```python
from build123d import *

# Parameters (mm, degrees)
SKETCH1_R           = 80
SKETCH1_R_2         = 1.1
SKETCH1_R_3         = 3.7
BOSS_EXTRUDE2_DEPTH = 3.175


with BuildPart() as part:
    # Sketch1 → Boss-Extrude2 (new body)
    with BuildSketch(Plane.XY):
        Circle(SKETCH1_R)
        with Locations((58.725568667, 44.315554285)):
            Circle(SKETCH1_R_2, mode=Mode.SUBTRACT)
        with Locations((67.741180127, 28.700057175)):
            Circle(SKETCH1_R_2, mode=Mode.SUBTRACT)
        with Locations((64.735398933, 37.375)):
            Circle(SKETCH1_R_2, mode=Mode.SUBTRACT)
        with Locations((50.050625842, 41.309773091)):
            Circle(SKETCH1_R_2, mode=Mode.SUBTRACT)
        with Locations((52.125683017, 19.684445715)):
            Circle(SKETCH1_R_2, mode=Mode.SUBTRACT)
        with Locations((43.110071557, 35.299942825)):
            Circle(SKETCH1_R_2, mode=Mode.SUBTRACT)
        with Locations((60.800625842, 22.690226909)):
            Circle(SKETCH1_R_2, mode=Mode.SUBTRACT)
        with Locations((46.115852752, 26.625)):
            Circle(SKETCH1_R_2, mode=Mode.SUBTRACT)
        with Locations((55.425625842, 32)):
            Circle(SKETCH1_R_3, mode=Mode.SUBTRACT)
        with Locations((-10.75, 64)):
            Circle(SKETCH1_R_2, mode=Mode.SUBTRACT)
        with Locations((-9.01561146, 73.01561146)):
            Circle(SKETCH1_R_2, mode=Mode.SUBTRACT)
        with Locations((9.01561146, 73.01561146)):
            Circle(SKETCH1_R_2, mode=Mode.SUBTRACT)
        with Locations((9.01561146, 54.98438854)):
            Circle(SKETCH1_R_2, mode=Mode.SUBTRACT)
        with Locations((-9.01561146, 54.98438854)):
            Circle(SKETCH1_R_2, mode=Mode.SUBTRACT)
        with Locations((0, 74.75)):
            Circle(SKETCH1_R_2, mode=Mode.SUBTRACT)
        with Locations((10.75, 64)):
            Circle(SKETCH1_R_2, mode=Mode.SUBTRACT)
        with Locations((0, 53.25)):
            Circle(SKETCH1_R_2, mode=Mode.SUBTRACT)
        with Locations((0, 64)):
            Circle(SKETCH1_R_3, mode=Mode.SUBTRACT)
        with Locations((67.741180127, -28.700057175)):
            Circle(SKETCH1_R_2, mode=Mode.SUBTRACT)
        with Locations((58.725568667, -44.315554285)):
            Circle(SKETCH1_R_2, mode=Mode.SUBTRACT)
        with Locations((64.735398933, -37.375)):
            Circle(SKETCH1_R_2, mode=Mode.SUBTRACT)
        with Locations((60.800625842, -22.690226909)):
            Circle(SKETCH1_R_2, mode=Mode.SUBTRACT)
        with Locations((43.110071557, -35.299942825)):
            Circle(SKETCH1_R_2, mode=Mode.SUBTRACT)
        with Locations((52.125683017, -19.684445715)):
            Circle(SKETCH1_R_2, mode=Mode.SUBTRACT)
        with Locations((50.050625842, -41.309773091)):
            Circle(SKETCH1_R_2, mode=Mode.SUBTRACT)
        with Locations((46.115852752, -26.625)):
            Circle(SKETCH1_R_2, mode=Mode.SUBTRACT)
        with Locations((55.425625842, -32)):
            Circle(SKETCH1_R_3, mode=Mode.SUBTRACT)
        with Locations((9.01561146, -73.01561146)):
            Circle(SKETCH1_R_2, mode=Mode.SUBTRACT)
        with Locations((-9.01561146, -73.01561146)):
            Circle(SKETCH1_R_2, mode=Mode.SUBTRACT)
        with Locations((0, -74.75)):
            Circle(SKETCH1_R_2, mode=Mode.SUBTRACT)
        with Locations((10.75, -64)):
            Circle(SKETCH1_R_2, mode=Mode.SUBTRACT)
        with Locations((-9.01561146, -54.98438854)):
            Circle(SKETCH1_R_2, mode=Mode.SUBTRACT)
        with Locations((9.01561146, -54.98438854)):
            Circle(SKETCH1_R_2, mode=Mode.SUBTRACT)
        with Locations((-10.75, -64)):
            Circle(SKETCH1_R_2, mode=Mode.SUBTRACT)
        with Locations((0, -53.25)):
            Circle(SKETCH1_R_2, mode=Mode.SUBTRACT)
        with Locations((0, -64)):
            Circle(SKETCH1_R_3, mode=Mode.SUBTRACT)
        with Locations((-58.725568667, -44.315554285)):
            Circle(SKETCH1_R_2, mode=Mode.SUBTRACT)
        with Locations((-67.741180127, -28.700057175)):
            Circle(SKETCH1_R_2, mode=Mode.SUBTRACT)
        with Locations((-64.735398933, -37.375)):
            Circle(SKETCH1_R_2, mode=Mode.SUBTRACT)
        with Locations((-50.050625842, -41.309773091)):
            Circle(SKETCH1_R_2, mode=Mode.SUBTRACT)
        with Locations((-52.125683017, -19.684445715)):
            Circle(SKETCH1_R_2, mode=Mode.SUBTRACT)
        with Locations((-43.110071557, -35.299942825)):
            Circle(SKETCH1_R_2, mode=Mode.SUBTRACT)
        with Locations((-60.800625842, -22.690226909)):
            Circle(SKETCH1_R_2, mode=Mode.SUBTRACT)
        with Locations((-46.115852752, -26.625)):
            Circle(SKETCH1_R_2, mode=Mode.SUBTRACT)
        with Locations((-55.425625842, -32)):
            Circle(SKETCH1_R_3, mode=Mode.SUBTRACT)
        with Locations((-67.741180127, 28.700057175)):
            Circle(SKETCH1_R_2, mode=Mode.SUBTRACT)
        with Locations((-58.725568667, 44.315554285)):
            Circle(SKETCH1_R_2, mode=Mode.SUBTRACT)
        with Locations((-64.735398933, 37.375)):
            Circle(SKETCH1_R_2, mode=Mode.SUBTRACT)
        with Locations((-60.800625842, 22.690226909)):
            Circle(SKETCH1_R_2, mode=Mode.SUBTRACT)
        with Locations((-43.110071557, 35.299942825)):
            Circle(SKETCH1_R_2, mode=Mode.SUBTRACT)
        with Locations((-52.125683017, 19.684445715)):
            Circle(SKETCH1_R_2, mode=Mode.SUBTRACT)
        with Locations((-50.050625842, 41.309773091)):
            Circle(SKETCH1_R_2, mode=Mode.SUBTRACT)
        with Locations((-46.115852752, 26.625)):
            Circle(SKETCH1_R_2, mode=Mode.SUBTRACT)
        with Locations((-55.425625842, 32)):
            Circle(SKETCH1_R_3, mode=Mode.SUBTRACT)
    extrude(amount=BOSS_EXTRUDE2_DEPTH)


solid = part.part
```
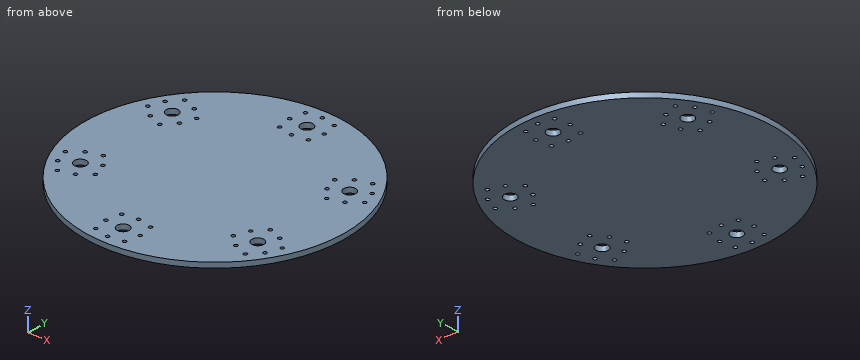
Source: CAD feature listing. Evaluate the final solid. Frame: model axes, mm. Round coordinates to 2 decimals unless told otherwise and drop trailing zeros. Order: outer loops, then holes, each group sorted by start corner. A loop starts at its lowest first (then second) coordinate and runs counter-clockwise, first axis right, second up. Notation, with made-up numbers: (20.25, 48) -> (36.25, 48) arc R20 ccw to (36.25, 75) -> close; hole circle Ø7 at (84.25, -28.75). An arc over 180 degrees is marked (long way). One line per item, written item: value. Start each with the question number.
Q1. Section query C-C (x = 24.5). Return the cut outline in (y, z) (3 decimals).
Q2. Section query B-B (x = -29.5). Return the cut outline in (y, z) (3 decimals).
Q3. Section query A-A (z = 0.65). Give the number of separate pieces and of enclosed holes in the cut face, plus the area to 3 significant figures.
Q4. Material intervals for probe 1 along Y at (x, z) = (-10.75, 1.1); probe 2 along Y at (x, z) = (-43.5, 0.35); probe 3 along X at (y, z) = (44, 2.4), sorted ascending.
Findings below:
1. outline: (-76.156, 0) -> (76.156, 0) -> (76.156, 3.175) -> (-76.156, 3.175) -> close
2. outline: (-74.362, 0) -> (74.362, 0) -> (74.362, 3.175) -> (-74.362, 3.175) -> close
3. separate pieces: 1
3. enclosed holes: 54
3. area: 19,700 mm²
4. probe 1: -79.27 to -65.1, -62.9 to 62.9, 65.1 to 79.27
4. probe 2: -67.14 to -36.33, -34.27 to 34.27, 36.33 to 67.14
4. probe 3: -66.81 to -59.78, -57.67 to 57.67, 59.78 to 66.81
